```python
from build123d import *

# Parameters (mm, degrees)
EXTRUDE_1_OUTLINE_W = 563.7
EXTRUDE_1_OUTLINE_H = 348.4
EXTRUDE_1_DEPTH     = 15
SKETCH_3_W          = 524
SKETCH_3_H          = 290
CUT_EXTRUDE_1_DEPTH = 70
SKETCH_4_W          = 10
SKETCH_4_H          = 348.4
EXTRUDE_2_DEPTH     = 15
SKETCH_5_W          = 583.7
SKETCH_5_H          = 20
EXTRUDE_3_DEPTH     = 15
SKETCH_6_W          = 10
SKETCH_6_H          = 224
CUT_EXTRUDE_2_DEPTH = 8
SKETCH_7_R          = 5
CUT_EXTRUDE_3_DEPTH = 10


# Read off the part's stored shape, not the designer's step: 填料-伸長1
with BuildPart() as part:
    # 填料-伸長1 outline → 填料-伸長1 (new body)
    with BuildSketch(Plane.XY):
        with Locations((83.50571914, 42.111680092)):
            Rectangle(EXTRUDE_1_OUTLINE_W, EXTRUDE_1_OUTLINE_H)
    extrude(amount=EXTRUDE_1_DEPTH)

    # 草圖3 → 除料-伸長1 (cut)
    with BuildSketch(Plane.XY.offset(15)):
        with Locations((83.50571914, 31.911680092)):
            Rectangle(SKETCH_3_W, SKETCH_3_H)
    extrude(amount=-CUT_EXTRUDE_1_DEPTH, mode=Mode.SUBTRACT)

    # 草圖4 → 填料-伸長2 (add)
    with BuildSketch(Plane.XY.offset(15)):
        with Locations((-203.34428086, 42.111680092)):
            Rectangle(SKETCH_4_W, SKETCH_4_H)
        with Locations((370.35571914, 42.111680092)):
            Rectangle(SKETCH_4_W, SKETCH_4_H)
    extrude(amount=-EXTRUDE_2_DEPTH)

    # 草圖5 → 填料-伸長3 (add)
    with BuildSketch(Plane.XY.offset(15)):
        with Locations((83.50571914, -142.088319908)):
            Rectangle(SKETCH_5_W, SKETCH_5_H)
    extrude(amount=-EXTRUDE_3_DEPTH)

    # 草圖6 → 除料-伸長2 (cut)
    with BuildSketch(Plane.XY.offset(15)):
        Polygon((364.50571914, -132.088319908), (364.50571914, 101.911680092), (354.50571914, 101.911680092), (354.50571914, -122.088319908), (354.50571914, -132.088319908), align=None)
        with BuildLine():
            Line((354.50571914, -132.088319908), (354.50571914, -122.088319908))
            Line((354.50571914, -122.088319908), (93.50571914, -122.088319908))
            Line((93.50571914, -122.088319908), (73.50571914, -122.088319908))
            Line((73.50571914, -122.088319908), (-187.49428086, -122.088319908))
            Line((-187.49428086, -122.088319908), (-197.49428086, -122.088319908))
            Line((-197.49428086, -122.088319908), (-197.49428086, -132.088319908))
            Line((-197.49428086, -132.088319908), (73.50571914, -132.088319908))
            Line((73.50571914, -132.088319908), (73.50571914, -139.088319908))
            ThreePointArc((73.50571914, -139.088319908), (74.384398796, -141.209640251), (76.50571914, -142.088319908))
            Line((76.50571914, -142.088319908), (90.50571914, -142.088319908))
            ThreePointArc((90.50571914, -142.088319908), (92.627039483, -141.209640251), (93.50571914, -139.088319908))
            Line((93.50571914, -139.088319908), (93.50571914, -132.088319908))
            Line((93.50571914, -132.088319908), (354.50571914, -132.088319908))
        make_face()
        with Locations((-192.49428086, -10.088319908)):
            Rectangle(SKETCH_6_W, SKETCH_6_H)
    extrude(amount=-CUT_EXTRUDE_2_DEPTH, mode=Mode.SUBTRACT)

    # 草圖7 → 除料-伸長3 (cut)
    with BuildSketch(Plane.XY.offset(7)):
        with Locations((83.50571914, -132.588319908)):
            Circle(SKETCH_7_R)
    extrude(amount=-CUT_EXTRUDE_3_DEPTH, mode=Mode.SUBTRACT)


solid = part.part
```
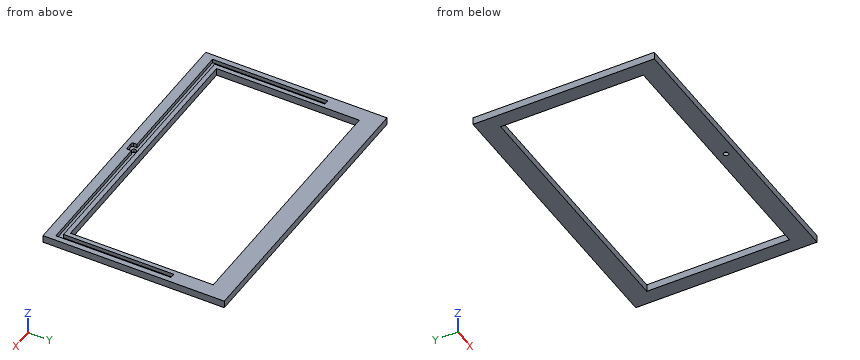
Source: CAD feature listing. Evaluate the final solid. Frame: model axes, mm. Give positions to 0.01 mm unless a question says otherwise; leave off trailing zeros. Loops run counter-clockwise (first coordinate to the right, second up) from the corner with the lowest first, then second, coordinate; pieces in that order, holes last. Notation, with made-up numbers: (-10.75, 73) -> (29.25, 73) arc R26 ccw to (29.25, 101) -> close; hole circle Ø2 at (-20.75, -34). An arc over 180 degrees is marked (long way). Put each result on its own line as item: value. Start each with the question number.
1) Cut plane D-D (y = -14). Return loops of the section in (x, z), then the cut area to 4 significant figures.
2) Cut plane C-C (z = 10.25). Return loops of the section in (x, y), then the cut area to 3 significant figures.
3) Material intervals for probe 1 along Y at (x, z) = (109, 13.75); probe 2 along X at (y, z) = (-86, 10.25); probe 3 along X at (y, z) = (44.5, 2.75), sorted ascending.
4) Contact query for a flat-ended pin moving along its axis: P1, Ø11.5, axis at x = 83.51, y = -132.59, coming from the +Z side. Output: stop coordinate, or through.
5) Cut plane A-A (x = -131). Return loops of the section in (y, z), then the cut area to 3 significant figures.
6) Cut plane B-B (y = 119). Return loops of the section in (x, z), then the cut area to 4 significant figures.
Results are:
1. outline: (-208.34, 0) -> (-178.49, 0) -> (-178.49, 15) -> (-187.49, 15) -> (-187.49, 7) -> (-197.49, 7) -> (-197.49, 15) -> (-208.34, 15) -> close; (345.51, 0) -> (375.36, 0) -> (375.36, 15) -> (364.51, 15) -> (364.51, 7) -> (354.51, 7) -> (354.51, 15) -> (345.51, 15) -> close
1. area: 735.5 mm2
2. outline: (-208.34, -152.09) -> (375.36, -152.09) -> (375.36, 216.31) -> (-208.34, 216.31) -> close; hole (-197.49, -132.09) -> (73.51, -132.09) -> (73.51, -139.09) arc R3 ccw to (76.51, -142.09) -> (90.51, -142.09) arc R3 ccw to (93.51, -139.09) -> (93.51, -132.09) -> (364.51, -132.09) -> (364.51, 101.91) -> (354.51, 101.91) -> (354.51, -122.09) -> (-187.49, -122.09) -> (-187.49, 101.91) -> (-197.49, 101.91) -> close; hole (-178.49, -113.09) -> (345.51, -113.09) -> (345.51, 176.91) -> (-178.49, 176.91) -> close
2. area: 52,800 mm2
3. probe 1: y = -152.09 to -132.09, -122.09 to -113.09, 176.91 to 216.31
3. probe 2: x = -208.34 to -197.49, -187.49 to -178.49, 345.51 to 354.51, 364.51 to 375.36
3. probe 3: x = -208.34 to -178.49, 345.51 to 375.36
4. P1: stops at z = 7
5. outline: (-152.09, 0) -> (-113.09, 0) -> (-113.09, 15) -> (-122.09, 15) -> (-122.09, 7) -> (-132.09, 7) -> (-132.09, 15) -> (-152.09, 15) -> close; (176.91, 0) -> (216.31, 0) -> (216.31, 15) -> (176.91, 15) -> close
5. area: 1,100 mm2
6. outline: (-208.34, 0) -> (-178.49, 0) -> (-178.49, 15) -> (-208.34, 15) -> close; (345.51, 0) -> (375.36, 0) -> (375.36, 15) -> (345.51, 15) -> close
6. area: 895.5 mm2
